Input: dimensioned drawing with shaded views. Units: mm. Origin: part minimum x, y, z. A direction names the side the tool comes from. Give positions to 0.01 mm unless a question says otherwise; leave off trailing zeros. Write each loop counter-clockwise with the first axis right and the second up, starting at its lowest first coordinate (ties: lowest second). Pieces come first, ordered by that corner, then holes.
Q1. Section C-C (y = 15.5). Return the cut outline in (x, z) (1 decimal).
Q2. Mould query, pull axis X, two halves, no side actions, for the marked faces 1, 2 and 3. Classes: +X half, -X half, draft (parallel to the pull), parting line (faces both ways), or undercut.
Q3. Section A-A (x = 22). Return the cut outline in (y, z), plus the area to 3 significant figures.
Q4. Line query: line 1 (X direction, y = 4, z = 43.5) (1 decimal); line 2 (Z direction, x = 68.5, y = 12.5). Output: solid intervals per line, ascending.
Q5. Section B-B (z = 46.5). Return the cut outline in (x, y) (1 decimal), plus the area to 3 significant figures.
Q6. Reachability of the marked faces 4 and 5 from +Z, -Z, +X, -X, +Y, -Y: full face, straight path, thin tool, end or side. Return the list, or none.
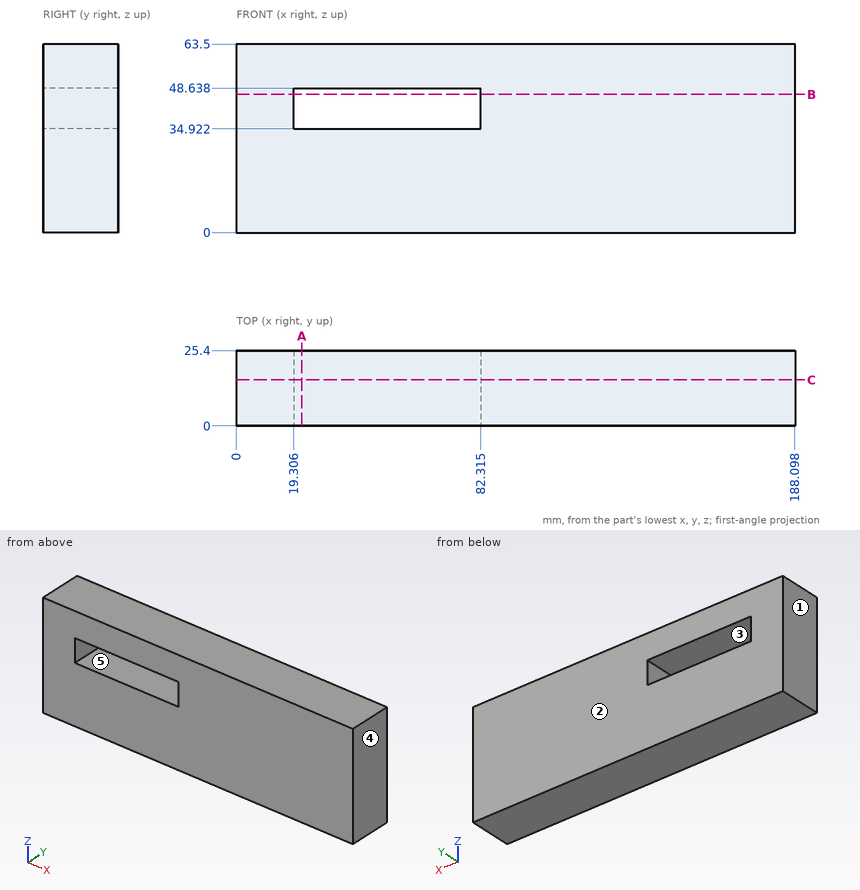
Computed:
1. outline: (0, 0) - (188.1, 0) - (188.1, 63.5) - (0, 63.5) - close; hole (19.3, 34.9) - (82.3, 34.9) - (82.3, 48.6) - (19.3, 48.6) - close
2. face 1: -X half
2. face 2: draft
2. face 3: undercut
3. outline: (0, 0) - (25.4, 0) - (25.4, 34.92) - (0, 34.92) - close; (0, 48.64) - (25.4, 48.64) - (25.4, 63.5) - (0, 63.5) - close
3. area: 1,260 mm2
4. line 1: x = 0 to 19.3, 82.3 to 188.1
4. line 2: z = 0 to 34.92, 48.64 to 63.5
5. outline: (0, 0) - (19.3, 0) - (19.3, 25.4) - (0, 25.4) - close; (82.3, 0) - (188.1, 0) - (188.1, 25.4) - (82.3, 25.4) - close
5. area: 3,180 mm2
6. face 4: +Z, -Z, +X, +Y, -Y
6. face 5: +Y, -Y
